Geometry check sheet. Reference: the model listing, model coordinates, mm. A direction names the side the tool comes from. Round coordinates to 2 decimals unless told otherwise and drop trailing zeros. Order: outer loops, then holes, each group sorted by start corner. A loop starts at its lowest first (then second) coordinate and runs counter-clockwise, first axis right, second up.
(1) Go/stop test with flat-tipped pins: pin 1 (0.6 mm diameter, centred on x = 34, y = 47.5, fed in from +Z); pin 2 (4 mm diameter, centred on x = 19.5, y = 18, fed in from -Z); pin 3 (1.4 mm diameter, centred on x = 12, y = 2.5, fed in from +Z). Record where each tip stops, or that it passes through.
(2) Sectioned sample at A-A (z = 3.5). Record the boundary of the cut face in (x, y), plus the area to 4 significant figures.
(3) Set-up check for faces 4 (the face through (6.24, 11.13, 7.64)), 5 (the face through (22, 34, 26.85)), 6 (the face through (18.69, 17.1, 17.85)): record each of +Z, -Z, +X, -X, +Y, -Y from which the full face is reachable in a straight line by a thin tool's end or side.
(4) Release check for a two-part mould opening along Y. For faces 1 (the face through (13, 19, 40)), 2 (the face through (-2.748, -1.396, 19.72)), 3 (the face through (30.352, 40.558, 33.51)) record: +Y half, -Y half, draft (parallel to the pull), parting line (faces both ways), or undercut.
(5) Sectioned sample at B-B (y = 25). Record the boundary of the cut face in (x, z).
(6) Material ranges on line 1 along X through (y, z) = (-0.6, 10); line 2 along Y through (x, z) = (26.5, 38.5); line 3 along X through (y, z) = (-1.2, 10), recorded low to high.
from build123d import *

# Parameters (mm, degrees)
BOSS_EXTRUDE1_DEPTH      = 40
SKETCH2_R                = 1.25
SKETCH2_R_2              = 1.5
SKETCH2_W                = 9
SKETCH2_H                = 9
SKETCH2_W_2              = 15.5
SKETCH2_H_2              = 7
CUT_EXTRUDE2_DEPTH       = 5
SKETCH4_W                = 7
SKETCH4_H                = 4
SKETCH4_H_2              = 2
BOSS_EXTRUDE2_DEPTH      = 5.5
SKETCH6_W                = 7
SKETCH6_H                = 2
BOSS_EXTRUDE3_DEPTH      = 7.5
BOSS_EXTRUDE4_DEPTH      = 3
BOSS_EXTRUDE4_DEPTH_BACK = 2
SKETCH10_W               = 1.5
SKETCH10_H               = 10
SKETCH10_W_2             = 10
SKETCH10_H_2             = 1.5
BOSS_EXTRUDE6_DEPTH      = 1.6
SKETCH5_R                = 1.6
CUT_EXTRUDE3_DEPTH       = 10
FILLET1_R                = 2


with BuildPart() as part:
    # Sketch1 → Boss-Extrude1 (new body)
    with BuildSketch(Plane.XY):
        Polygon((0, 0), (37.395775338, 53.406702009), (35.347895227, 54.8406431), (-4.802455317, -2.5), (0, -2.5), (30, -2.5), (30, 0), align=None)
    extrude(amount=BOSS_EXTRUDE1_DEPTH)

    # Sketch2 → Cut-Extrude2 (cut)
    with BuildSketch(Plane(origin=(-2.047880111, 1.433941091, 0), x_dir=(0, 0, 1), z_dir=(-0.8191520442889935, 0.5735764363510438, 0))):
        Polygon((26.85, 42.812544683), (32.75, 42.812544683), (32.75, 58.312544683), (7.25, 58.312544683), (7.25, 42.812544683), (12.85, 42.812544683), (12.85, 38.812544683), (26.85, 38.812544683), align=None)
        with Locations(Location((8.7, 39.047544683, 0), (0, 0, 270))):
            Circle(SKETCH2_R)
        with Locations(Location((31.3, 39.047544683, 0), (0, 0, 270))):
            Circle(SKETCH2_R)
        with Locations(Location((8.7, 61.577544683, 0), (0, 0, 270))):
            Circle(SKETCH2_R)
        with Locations(Location((31.3, 61.577544683, 0), (0, 0, 270))):
            Circle(SKETCH2_R)
        with Locations(Location((10.8, 25.197544683, 0), (0, 0, 270))):
            Circle(SKETCH2_R_2)
        with Locations(Location((24.8, 25.197544683, 0), (0, 0, 270))):
            Circle(SKETCH2_R_2)
        with Locations((20, 16.197544683)):
            Rectangle(SKETCH2_W, SKETCH2_H)
        with Locations((7.75, 16.197544683)):
            Rectangle(SKETCH2_W_2, SKETCH2_H_2)
    extrude(amount=-CUT_EXTRUDE2_DEPTH, mode=Mode.SUBTRACT)

    # Sketch4 → Boss-Extrude2 (add)
    with BuildSketch(Plane(origin=(0, 0, 0), x_dir=(0, 0, -1), z_dir=(0.8191520442889932, -0.5735764363510439, 0))):
        with Locations((-17.8, 24.697544683)):
            Rectangle(SKETCH4_W, SKETCH4_H)
        with Locations((-20, 9.697544683)):
            Rectangle(SKETCH4_W, SKETCH4_H_2)
    extrude(amount=BOSS_EXTRUDE2_DEPTH)

    # Sketch6 → Boss-Extrude3 (add)
    with BuildSketch(Plane(origin=(0, 0, 0), x_dir=(0, 0, -1), z_dir=(0.8191520442889932, -0.5735764363510439, 0))):
        with Locations((-17.8, 27.697544683)):
            Rectangle(SKETCH6_W, SKETCH6_H)
        with Locations((-20, 7.697544683)):
            Rectangle(SKETCH6_W, SKETCH6_H)
    extrude(amount=BOSS_EXTRUDE3_DEPTH)

    # Sketch8 → Boss-Extrude4 (add, two sides: drawn at the far end of the back side and taken through both)
    with BuildSketch(Plane(origin=(4.988706684, 7.124611507, 21.197544683), x_dir=(0.671010071662837, -0.4698463103929531, -0.5735764363510439), z_dir=(0.5735764363510439, 0.8191520442889935, 0)).offset(-BOSS_EXTRUDE4_DEPTH_BACK)):
        Polygon((8.838041271, -0.453819943), (4.823006216, -6.187884253), (6.461310305, -7.335037125), (10.476345359, -1.600972815), align=None)
    extrude(amount=BOSS_EXTRUDE4_DEPTH + BOSS_EXTRUDE4_DEPTH_BACK)

    # Sketch10 → Boss-Extrude6 (add)
    with BuildSketch(Plane(origin=(0, 0, 0), x_dir=(0, 0, -1), z_dir=(0.8191520442889934, -0.5735764363510439, 0))):
        with Locations((-33.5, 50.562544683)):
            Rectangle(SKETCH10_W, SKETCH10_H)
        with Locations((-6.5, 50.562544683)):
            Rectangle(SKETCH10_W, SKETCH10_H)
        with Locations((-20, 59.062544683)):
            Rectangle(SKETCH10_W_2, SKETCH10_H_2)
    extrude(amount=BOSS_EXTRUDE6_DEPTH)

    # Sketch5 → Cut-Extrude3 (cut)
    with BuildSketch(Plane(origin=(0, 0, 0), x_dir=(1, 0, 0), z_dir=(0, 1, 0))):
        with Locations(Location((15, -10, 0), (0, 0, 270))):
            Circle(SKETCH5_R)
        with Locations(Location((15, -30, 0), (0, 0, 270))):
            Circle(SKETCH5_R)
    extrude(amount=-CUT_EXTRUDE3_DEPTH, mode=Mode.SUBTRACT)

    # Fillet1
    # the kernel refuses this fillet: 2 mm, written as the material it adds along each edge
    with BuildSketch(Plane(origin=(0, 0, 0), x_dir=(0.5735764363510439, 0.8191520442889934, 0), z_dir=(0, 0, 1))) as fillet1_piece_1:
        with BuildLine():
            CenterArc((FILLET1_R * 1.92098212697, -FILLET1_R), FILLET1_R, 90, 125)
            Line((FILLET1_R * 1.10183008268, -FILLET1_R * 1.57357643635), (0, 0))
            Line((0, 0), (FILLET1_R * 1.92098212697, 0))
        make_face()
    extrude(amount=40)
    with BuildSketch(Plane(origin=(9.82374381, 18.388377129, 24.5), x_dir=(-0.5735764363510438, -0.8191520442889935, 0), z_dir=(0.8191520442889935, -0.5735764363510438, 0)), Plane(origin=(4.661555882, 11.016008731, 24.5), x_dir=(0, 0, -1), z_dir=(0.8191520442889935, -0.5735764363510438, 0))) as fillet1_piece_2:
        with BuildLine():
            CenterArc((FILLET1_R, FILLET1_R), FILLET1_R, 180, 90)
            Line((0, FILLET1_R), (0, 0))
            Line((0, 0), (FILLET1_R, 0))
        make_face()
    extrude(amount=2.5)
    with BuildSketch(Plane(origin=(4.661555882, 11.016008731, 15.5), x_dir=(0.5735764363510438, 0.8191520442889935, 7.105427357600794e-14), z_dir=(0.8191520442889935, -0.5735764363510438, 0))) as fillet1_piece_3:
        with BuildLine():
            CenterArc((2, 1.732050808), FILLET1_R, 180, 60)
            Line((0, 1.732050808), (0, 0))
            Line((0, 0), (1, 0))
        make_face()
    extrude(amount=2.5)
    with BuildSketch(Plane(origin=(9.82374381, 18.388377129, 15.5), x_dir=(0, 0, 1), z_dir=(0.8191520442889935, -0.5735764363510438, 0))) as fillet1_piece_4:
        with BuildLine():
            CenterArc((1.732050808, 2), FILLET1_R, 210, 60)
            Line((0, 1), (0, 0))
            Line((0, 0), (1.732050808, 0))
        make_face()
    extrude(amount=2.5)
    # the kernel refuses this fillet: 2 mm, written as the material it takes off along each edge
    with BuildSketch(Plane(origin=(41.491535559, 50.538819828, 40), x_dir=(0, 0, -1), z_dir=(-0.8191520442889935, 0.5735764363510437, 0)), Plane(origin=(30, -7.5, 0), x_dir=(-1, 0, 0), z_dir=(0, 1, 0)), Plane(origin=(41.491535559, 50.538819828, 0), x_dir=(-0.5735764363510438, -0.8191520442889935, 0), z_dir=(-0.8191520442889935, 0.5735764363510437, 0))) as fillet1_2_piece_1:
        with BuildLine():
            CenterArc((FILLET1_R, FILLET1_R), FILLET1_R, 180, 90)
            Line((0, FILLET1_R), (0, 0))
            Line((0, 0), (FILLET1_R, 0))
        make_face()
    extrude(amount=12.5, mode=Mode.SUBTRACT)
    with BuildSketch(Plane(origin=(-4.802455317, -2.5, -9.604910635), x_dir=(1, 0, 0), z_dir=(0, 0, 1))) as fillet1_2_piece_2:
        with BuildLine():
            CenterArc((FILLET1_R * 1.92098212697, FILLET1_R), FILLET1_R, 145, 125)
            Line((FILLET1_R * 1.10183008268, FILLET1_R * 1.57357643635), (0, 0))
            Line((0, 0), (FILLET1_R * 1.92098212697, 0))
        make_face()
    extrude(amount=59.20982127, mode=Mode.SUBTRACT)
    with BuildSketch(Plane(origin=(30, -7.5, 40), x_dir=(-1, 0, 0), z_dir=(0, 1, 0))) as fillet1_2_piece_3:
        with BuildLine():
            CenterArc((FILLET1_R, -FILLET1_R), FILLET1_R, 90, 90)
            Line((0, -FILLET1_R), (0, 0))
            Line((0, 0), (FILLET1_R, 0))
        make_face()
    extrude(amount=12.5, mode=Mode.SUBTRACT)


solid = part.part
Answer below:
1. pin 1: stops at z = 25
1. pin 2: stops at z = 14.3
1. pin 3: stops at z = 23.5
2. outline: (-2.6, 0.65) arc R2 ccw to (-0.96, -2.5) - (30, -2.5) - (30, 0) - (3.84, 0) arc R2 cw to (2.2, 3.15) - (7.28, 10.4) - (5.24, 11.84) - close; (9.25, 17.57) - (11.3, 16.14) - (37.4, 53.41) - (35.35, 54.84) - close
2. area: 232.5 mm2
3. face 4: -Z, +X, +Y
3. face 5: +X, +Y
3. face 6: +Z, -Z
4. face 1: draft
4. face 2: parting line
4. face 3: undercut
5. outline: (14.45, 0) - (17.51, 0) - (17.51, 40) - (14.45, 40) - close
6. line 1: x = -2.96 to 13.4, 16.6 to 30
6. line 2: y = -2.5 to 0, 37.85 to 42.2
6. line 3: x = -2.83 to 13.4, 16.6 to 30
